Model file for the job. Use its own axes, mm. Face numbers are marked on the shaded views. Coordinates: 2 decimals unless noted, no trailing zeros. Write each loop counter-clockwise with the first axis right and the second up, starting at its lowest first coordinate (ties: lowest second). Pieces come first, ordered by that corner, then holes.
Q1. Band-saw the part on C-C, the plane x = -215. Write the cut outline in (y, z).
Q2. Pull direction X, two halves, no side cores. Call the marked faces 1, 2 and 3: released by +X, released by -X, zero draft, split by the parting line, or undercut.
Q3. Pin check, flat tips, straight feed: P1, Ø2, axis at x = -154, z = 27, coming from the +Y side; P2, Ø3, axis at y = -32, z = 33.5, coming from the -X side; P3, Ø5, axis at x = -46, y = -2, coming from the +Z side; P4, Ø4, axis at x = -19, z = 32, coming from the -Y side. Stop position of each tip, or through.
Q4. Band-saw the part on D-D, the plane x = -269.5. Write the cut outline in (y, z), plus the area to 3 significant figures.
Q5. Band-saw the part on A-A, the plane z = 29.5. Write the cut outline in (x, y), plus the area to 3 significant figures.
Q6. Band-saw the part on B-B, the plane y = 7. Write the cut outline in (x, z).
Q7. Drill centre lines: probe 1 along Y at (x, z) = (-224, 41); probe 2 along X at (y, z) = (10, 41); probe 3 along X at (y, z) = (-30.5, 23.5). Where is each one in solid material? Low to high.
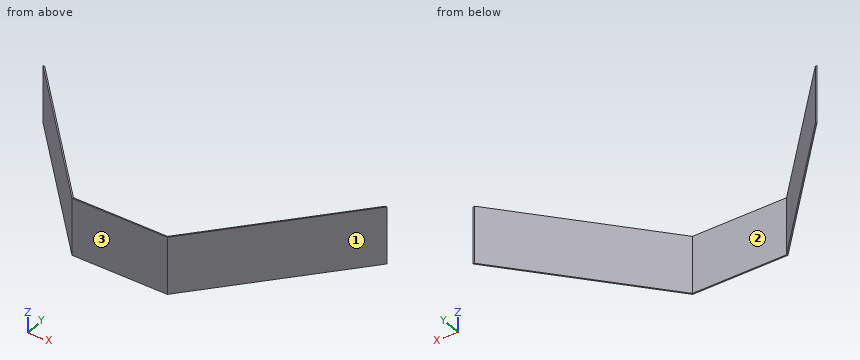
from build123d import *

# Parameters (mm, degrees)
BOSS_EXTRUDE1_DEPTH = 69.85
SHELL10_T           = -1.524


with BuildPart() as part:
    # Sketch1 → Boss-Extrude1 (new body)
    with BuildSketch(Plane.XY):
        Polygon((-374.797674419, 95.508430233), (37.952325581, 95.508430233), (-111.272674419, -69.591569767), (-225.572674419, -69.591569767), align=None)
    extrude(amount=BOSS_EXTRUDE1_DEPTH)

    # Shell10
    shell10_openings = [part.faces().sort_by_distance(p)[0] for p in [
        (-168.422674419, 12.958430233, 69.85),
        (-168.422674419, 12.958430233, 0),
        (-168.422674419, 95.508430233, 34.925),
    ]]
    offset(amount=SHELL10_T, openings=shell10_openings, kind=Kind.INTERSECTION)


solid = part.part
Answer sheet:
1. outline: (-69.59, 0) - (-68.07, 0) - (-68.07, 69.85) - (-69.59, 69.85) - close
2. face 1: released by +X
2. face 2: undercut
2. face 3: zero draft
3. P1: stops at y = -68.07
3. P2: stops at x = -260.91
3. P3: passes through
3. P4: stops at y = 30.28
4. outline: (-20.99, 0) - (-18.72, 0) - (-18.72, 69.85) - (-20.99, 69.85) - close
4. area: 159 mm2
5. outline: (-374.8, 95.51) - (-225.57, -69.59) - (-111.27, -69.59) - (37.95, 95.51) - (35.9, 95.51) - (-111.95, -68.07) - (-224.9, -68.07) - (-372.74, 95.51) - close
5. area: 848 mm2
6. outline: (-294.8, 0) - (-292.75, 0) - (-292.75, 69.85) - (-294.8, 69.85) - close; (-44.1, 0) - (-42.05, 0) - (-42.05, 69.85) - (-44.1, 69.85) - close
7. probe 1: y = -69.59 to -68.07
7. probe 2: x = -297.51 to -295.46, -41.39 to -39.33
7. probe 3: x = -260.91 to -258.85, -77.99 to -75.94
